```python
from build123d import *

# Parameters (mm, degrees)
ESQUISSE1_R      = 3
ESQUISSE1_R_2    = 1.5
ESQUISSE1_W      = 17
ESQUISSE1_H      = 192
EXTRUSION1_DEPTH = 2
ESQUISSE3_R      = 1.5
ESQUISSE3_R_2    = 2
EXTRUSION2_DEPTH = 10


with BuildPart() as part:
    # Esquisse1 → Extrusion1 (new body)
    with BuildSketch(Plane.XY):
        Polygon((1.932476129, -483.38221942), (106.932476129, -483.38221942), (106.932476129, -207.38221942), (-23.067523871, -207.38221942), (-23.067523871, -468.38221942), (1.932476129, -468.38221942), align=None)
        with Locations((-16.067523871, -214.38221942)):
            Circle(ESQUISSE1_R, mode=Mode.SUBTRACT)
        with Locations(Location((8.932476129, -468.38221942, 0), (0, 0, 180))):
            Circle(ESQUISSE1_R_2, mode=Mode.SUBTRACT)
        with Locations((10.932476129, -212.38221942)):
            Circle(ESQUISSE1_R_2, mode=Mode.SUBTRACT)
        with Locations(Location((8.932476129, -478.38221942, 0), (0, 0, 180))):
            Circle(ESQUISSE1_R_2, mode=Mode.SUBTRACT)
        with Locations((60.932476129, -268.88221942)):
            Circle(ESQUISSE1_R_2, mode=Mode.SUBTRACT)
        with Locations((29.932476129, -268.88221942)):
            Circle(ESQUISSE1_R_2, mode=Mode.SUBTRACT)
        with Locations((29.932476129, -237.88221942)):
            Circle(ESQUISSE1_R_2, mode=Mode.SUBTRACT)
        with Locations((60.932476129, -237.88221942)):
            Circle(ESQUISSE1_R_2, mode=Mode.SUBTRACT)
        with Locations((29.932476129, -253.38221942)):
            Circle(ESQUISSE1_R_2, mode=Mode.SUBTRACT)
        with Locations((60.932476129, -253.38221942)):
            Circle(ESQUISSE1_R_2, mode=Mode.SUBTRACT)
        with Locations((16.932476129, -222.38221942)):
            Circle(ESQUISSE1_R_2, mode=Mode.SUBTRACT)
        with Locations((72.932476129, -478.38221942)):
            Circle(ESQUISSE1_R_2, mode=Mode.SUBTRACT)
        with Locations((45.432476129, -253.38221942)):
            Circle(ESQUISSE1_R, mode=Mode.SUBTRACT)
        with Locations((66.932476129, -468.38221942)):
            Circle(ESQUISSE1_R_2, mode=Mode.SUBTRACT)
        with Locations((74.932476129, -222.38221942)):
            Circle(ESQUISSE1_R_2, mode=Mode.SUBTRACT)
        with Locations(Location((99.932476129, -214.38221942, 0), (0, 0, 180))):
            Circle(ESQUISSE1_R, mode=Mode.SUBTRACT)
        with Locations((74.932476129, -212.38221942)):
            Circle(ESQUISSE1_R_2, mode=Mode.SUBTRACT)
        with Locations(Location((-16.067523871, -458.38221942, 0), (0, 0, 180))):
            Circle(ESQUISSE1_R, mode=Mode.SUBTRACT)
        with Locations((99.932476129, -458.38221942)):
            Circle(ESQUISSE1_R, mode=Mode.SUBTRACT)
        with Locations((38.432476129, -370.88221942)):
            Rectangle(ESQUISSE1_W, ESQUISSE1_H, mode=Mode.SUBTRACT)
    extrude(amount=EXTRUSION1_DEPTH)

    # Esquisse3 → Extrusion2 (cut)
    with BuildSketch(Plane.XY.offset(2)):
        with Locations((-3.067523871, -237.38221942)):
            Circle(ESQUISSE3_R)
        with Locations((86.932476129, -237.38221942)):
            Circle(ESQUISSE3_R)
        with Locations((86.932476129, -437.38221942)):
            Circle(ESQUISSE3_R)
        with Locations((-3.067523871, -437.38221942)):
            Circle(ESQUISSE3_R)
        with Locations((-3.067523871, -337.38221942)):
            Circle(ESQUISSE3_R)
        with Locations((86.932476129, -337.38221942)):
            Circle(ESQUISSE3_R)
        with Locations((-3.067523871, -287.38221942)):
            Circle(ESQUISSE3_R)
        with Locations((86.932476129, -287.38221942)):
            Circle(ESQUISSE3_R)
        with Locations((-3.067523871, -387.38221942)):
            Circle(ESQUISSE3_R)
        with Locations((86.932476129, -387.38221942)):
            Circle(ESQUISSE3_R)
        with Locations((42.932476129, -473.38221942)):
            Circle(ESQUISSE3_R_2)
        with Locations((-18.067523871, -203.38221942)):
            Circle(ESQUISSE3_R)
        with Locations((101.932476129, -203.38221942)):
            Circle(ESQUISSE3_R)
        with Locations((-18.067523871, -387.38221942)):
            Circle(ESQUISSE3_R)
        with Locations((101.932476129, -387.38221942)):
            Circle(ESQUISSE3_R)
    extrude(amount=-EXTRUSION2_DEPTH, mode=Mode.SUBTRACT)


solid = part.part
```
Geometry: final body of the model. Coordinates: model frame, mm. Round coordinates to 2 decimals unless told otherwise and drop trailing zeros. Write each loop counter-clockwise with the first axis right and the second up, starting at its lowest first coordinate (ties: lowest second). Pieces come first, ordered by that corner, then holes. Notation, with made-up numbers: (89.25, 1) -> (136.25, 1) arc R25 ccw to (136.25, 26) -> close; hole circle Ø11 at (6.5, 62.25). An arc over 180 degrees is marked (long way). Use CSV: the item, a comma, the result in double quotes. Start each with the question number.
Q1. Section B-B (z = 1.3). Give the number of separate pieces and of enclosed holes in the cut face, plus the area to 3 significant figures.
Q2. Line query: L1, parallel to Y at x = -16, z = 1.05; L2, parallel to X at y = -305, z = 0.5; L3, parallel to Y at x = 39.5, z = 1.7. Output: solid intervals per line, ascending.
Q3. Section A-A (y = -433). Return loops of the section in (x, z).
Q4. Pull-direction query (X, two-part tool) for faces 1 (the face through (97.552, -460.208, 0.986)), 2 (the face through (55, -343, 2)); classes: pulls with the +X half, pulls with the -X half, needs draft (parallel to the pull), parting line crosses it, or undercut.
Q5. First-contact query: pin 1 Ø2.5 at (x, y) = (60.93, -237.88) entering from -Z. Flat tip, straight axial feed; report the tip coordinate or a pass-through.
Result sheet:
1,separate pieces,"1"
1,enclosed holes,"33"
1,area,"31,900 mm²"
2,L1,"-468.38 to -461.38, -455.38 to -217.38, -211.38 to -207.38"
2,L2,"-23.07 to 29.93, 46.93 to 106.93"
2,L3,"-483.38 to -466.88, -274.88 to -207.38"
3,outline,"(-23.07, 0) -> (29.93, 0) -> (29.93, 2) -> (-23.07, 2) -> close; (46.93, 0) -> (106.93, 0) -> (106.93, 2) -> (46.93, 2) -> close"
4,face 1,"undercut"
4,face 2,"needs draft"
5,pin 1,"through"
